Read the model definition and answer for the solid it produces. Units are mm, in the model's axes. A direction names the side the tool comes from. Round coordinates to 2 decimals unless told otherwise and drop trailing zeros. Order: outer loops, then holes, each group sorted by start corner. A loop starts at its lowest first (then second) coordinate and runs counter-clockwise, first axis right, second up. Notation, with made-up numbers: (69.25, -6.5) -> (113.25, -6.5) arc R6 ccw to (113.25, -0.5) -> close; hole circle Ø4 at (-19.5, 11.5). An arc over 180 degrees is marked (long way). Use a Markdown table: item, result. Add a question column.
1. The mould has two halves that part along Y. Classify faces 1 (the face through (14, -2, 0)), 2 (the face through (0, 0, 0)), 3 (the face through (-21, -11, 0)), 4 (the face through (-18.3, -4, 0)): +Y half, -Y half, draft (parallel to the pull), parting line (faces both ways), or undercut.
2. For faces 5 (the face through (-21, -9, -5.5)), 6 (the face through (0, -6, 8)), 7 (the face through (0, -7, -6)), determine the directions among +Z, -Z, +X, -X, +Y, -Y from which every point of the face is accessible in a straight line to the end or side of a thin tool.
3. Consider L1, parallel to X at y = -3, z = 3.25; L2, parallel to Z at x = -5, y = -5; L3, parallel to X at y = -10, z = 1. Determine where each line is inside the solid, lowest interval first. Write a range as [from, to].
4. Section C-C, the plane y = -9.5 is taken. Give the vertices of the cut face in (x, z).
5. Section A-A, the plane z = -1.5 is taken. Give the vertices of the cut face in (x, y).
6. Given pin 1 (1.9 mm diameter, centred on x = -19, z = 0.5, fed in from -Y); pin 2 (3 mm diameter, centred on y = -9, z = -0.5, fed in from -X), each flat-ended and moving along its own axis, determine where each tip first touches the part or whether it passes through.
7. Section B-B, the plane y = -4 is taken. Give the vertices of the cut face in (x, z).
8. Section D-D, the plane x = -2 is taken. Give the vertices of the cut face in (y, z), then the cut area to 3 significant figures.
```python
from build123d import *

# Parameters (mm, degrees)
SKETCH_1_W          = 44
SKETCH_1_H          = 16
EXTRUDE_1_DEPTH     = 2
SKETCH_2_W          = 44
SKETCH_2_H          = 16
SKETCH_2_W_2        = 40
SKETCH_2_H_2        = 12
EXTRUDE_2_DEPTH     = 10
SKETCH_3_W          = 5.5
SKETCH_3_H          = 4
CUT_EXTRUDE_1_DEPTH = 2
SKETCH_4_W          = 1.7
SKETCH_4_H          = 12
EXTRUDE_4_DEPTH     = 4.6
SKETCH_9_W          = 44
SKETCH_9_H          = 16
SKETCH_9_W_2        = 42
SKETCH_9_H_2        = 14
EXTRUDE_5_DEPTH     = 1
SKETCH_12_W         = 1
SKETCH_12_H         = 12
CUT_EXTRUDE_3_DEPTH = 5


with BuildPart() as part:
    # 草图1 → 凸台-拉伸1 (new body)
    with BuildSketch(Plane(origin=(0, 0, 0), x_dir=(1, 0, 0), z_dir=(0, 1, 0))):
        Rectangle(SKETCH_1_W, SKETCH_1_H)
    extrude(amount=-EXTRUDE_1_DEPTH)

    # 草图2 → 凸台-拉伸2 (add)
    with BuildSketch(Plane.XZ.offset(2)):
        Rectangle(SKETCH_2_W, SKETCH_2_H)
        Rectangle(SKETCH_2_W_2, SKETCH_2_H_2, mode=Mode.SUBTRACT)
    extrude(amount=EXTRUDE_2_DEPTH)

    # 草图3 → 切除-拉伸1 (cut)
    with BuildSketch(Plane.ZY.offset(22)):
        with Locations((2.75, -9)):
            Rectangle(SKETCH_3_W, SKETCH_3_H)
        with Locations((-2.75, -9)):
            Rectangle(SKETCH_3_W, SKETCH_3_H)
    extrude(amount=-CUT_EXTRUDE_1_DEPTH, mode=Mode.SUBTRACT)

    # 草图4 → 凸台-拉伸4 (add)
    with BuildSketch(Plane.XZ.offset(2)):
        with Locations((7.15, 0)):
            Rectangle(SKETCH_4_W, SKETCH_4_H)
        with Locations((-19.15, 0)):
            Rectangle(SKETCH_4_W, SKETCH_4_H)
        with Locations((-6, 0)):
            Rectangle(SKETCH_4_W, SKETCH_4_H)
    extrude(amount=EXTRUDE_4_DEPTH)

    # 草图9 → 凸台-拉伸5 (add)
    with BuildSketch(Plane.XZ.offset(12)):
        Rectangle(SKETCH_9_W, SKETCH_9_H)
        Rectangle(SKETCH_9_W_2, SKETCH_9_H_2, mode=Mode.SUBTRACT)
    extrude(amount=EXTRUDE_5_DEPTH)

    # 草图12 → 切除-拉伸3 (cut)
    with BuildSketch(Plane.XZ.offset(12)):
        with Locations((20.5, 0)):
            Rectangle(SKETCH_12_W, SKETCH_12_H)
    extrude(amount=-CUT_EXTRUDE_3_DEPTH, mode=Mode.SUBTRACT)


solid = part.part
```
Verdict:
| question | item | result |
|---|---|---|
| 1 | face 1 | -Y half |
| 1 | face 2 | +Y half |
| 1 | face 3 | undercut |
| 1 | face 4 | draft |
| 2 | face 5 | -X |
| 2 | face 6 | +Z, +X, -X, +Y, -Y |
| 2 | face 7 | -Y |
| 3 | L1 | x = [-22, -18.3], [-6.85, -5.15], [6.3, 8], [20, 22] |
| 3 | L2 | z = [-8, -6], [6, 8] |
| 3 | L3 | x = [21, 22] |
| 4 | outline | (-22, -8) -> (22, -8) -> (22, 8) -> (-22, 8) -> (-22, 5.5) -> (-20, 5.5) -> (-20, 6) -> (21, 6) -> (21, -6) -> (-20, -6) -> (-20, -5.5) -> (-22, -5.5) -> close |
| 5 | outline | (-22, -13) -> (-21, -13) -> (-21, -12) -> (-20, -12) -> (-20, -11) -> (-22, -11) -> close; (-22, -7) -> (-20, -7) -> (-20, -6.6) -> (-18.3, -6.6) -> (-18.3, -2) -> (-6.85, -2) -> (-6.85, -6.6) -> (-5.15, -6.6) -> (-5.15, -2) -> (6.3, -2) -> (6.3, -6.6) -> (8, -6.6) -> (8, -2) -> (20, -2) -> (20, -7) -> (21, -7) -> (21, -13) -> (22, -13) -> (22, 0) -> (-22, 0) -> close |
| 6 | pin 1 | stops at y = -6.6 |
| 6 | pin 2 | stops at x = 21 |
| 7 | outline | (-22, -8) -> (22, -8) -> (22, 8) -> (-22, 8) -> close; hole (-18.3, -6) -> (-6.85, -6) -> (-6.85, 6) -> (-18.3, 6) -> close; hole (-5.15, -6) -> (6.3, -6) -> (6.3, 6) -> (-5.15, 6) -> close; hole (8, -6) -> (20, -6) -> (20, 6) -> (8, 6) -> close |
| 8 | outline | (-13, -8) -> (0, -8) -> (0, 8) -> (-13, 8) -> (-13, 7) -> (-12, 7) -> (-12, 6) -> (-2, 6) -> (-2, -6) -> (-12, -6) -> (-12, -7) -> (-13, -7) -> close |
| 8 | area | 74.0 mm2 |
